Geometry: final body of the model. Coordinates: model frame, mm. Face numbers are marked on the shaded views. A direction names the side the tool comes from. Give positions to 0.01 mm unless a question says otherwise; leave off trailing zeros. Write each loop counter-clockwise with the first axis right and the second up, starting at its lowest first coordinate (ties: lowest second). Pieces come first, ordered by that corner, then holes. Notation, with made-up numbers: (2, 74) - (43, 74) arc R18 cw to (43, 98) - close; hole circle Ø8 at (46, 10.25). An arc over 180 degrees is marked (long way). Use CSV: the item, a comma, the result in double quotes. Start each with the question number.
(1) Section A-A on z = 1. Output: boundary loops of the cut face in (x, y), and give its area (3 significant figures).
(2) Reachability of the marked faces 5 and 6 from +Z, -Z, +X, -X, +Y, -Y: full face, straight path, thin tool, end or side. Return the list, or none.
(3) Section D-D on z = 6.25. Output: boundary loops of the cut face in (x, y), and give its area (3 significant figures).
(4) Draft query along Y for the marked faces 1, 2, 3 and 4. Return one class per face: released by +Y, released by -Y, zero draft, split by the parting line, or undercut.
(5) Line query: probe 1 along Y at (x, z) = (-20.5, 1.65); probe 2 along Y at (x, z) = (20.5, 7); probe 3 along Z at (x, y) = (16.5, 17.5). Output: solid intervals per line, ascending. Write a range as [from, to].
(6) Section C-C on y = 19.5. Output: boundary loops of the cut face in (x, z).
(7) First-contact query: pin 1 Ø4 at (x, y) = (-20.5, 19.5) entering from -Z; pin 2 Ø8.5 at (x, y) = (-20.5, 19.5) entering from +Z. Flat tips, straight axial feed; report the tip coordinate or a pass-through.
(8) Section B-B on x = 0. Output: boundary loops of the cut face in (y, z).
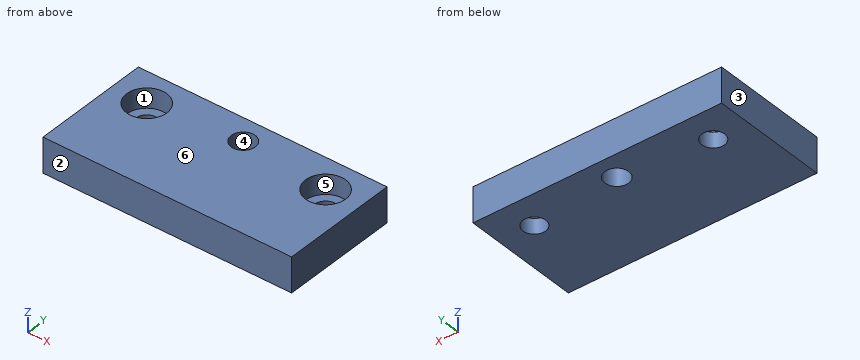
from build123d import *

# Parameters (mm, degrees)
F0_W     = 57
F0_H     = 27
F1_DEPTH = 8
F2_R     = 2.75
F2_R_2   = 2.6
F3_DEPTH = 9
F2_R_3   = 4.6
F4_DEPTH = 4.5


with BuildPart() as f1:
    # F0 (on Top) → F1 (new body)
    with BuildSketch(Plane.XY):
        with Locations((0, 13.5)):
            Rectangle(F0_W, F0_H)
    extrude(amount=F1_DEPTH)

    # F2 (on face) → F3 (cut)
    with BuildSketch(Plane.XY.offset(8)):
        with Locations((0, 21.5)):
            Circle(F2_R)
        with Locations((20.5, 19.5)):
            Circle(F2_R_2)
        with Locations((-20.5, 19.5)):
            Circle(F2_R_2)
    extrude(amount=-F3_DEPTH, mode=Mode.SUBTRACT)

    # F2 (on face) → F4 (cut)
    with BuildSketch(Plane.XY.offset(8)):
        with Locations((-20.5, 19.5)):
            Circle(F2_R_3)
        with Locations((-20.5, 19.5)):
            Circle(F2_R_2, mode=Mode.SUBTRACT)
        with Locations((20.5, 19.5)):
            Circle(F2_R_3)
        with Locations((20.5, 19.5)):
            Circle(F2_R_2, mode=Mode.SUBTRACT)
        with Locations((0, 21.5)):
            Circle(F2_R)
    extrude(amount=-F4_DEPTH, mode=Mode.SUBTRACT)


solid = f1.part
Check values:
1,outline,"(-28.5, 0) - (28.5, 0) - (28.5, 27) - (-28.5, 27) - close; hole circle Ø5.2 at (-20.5, 19.5); hole circle Ø5.5 at (0, 21.5); hole circle Ø5.2 at (20.5, 19.5)"
1,area,"1,470 mm²"
2,face 5,"+Z"
2,face 6,"+Z, +X, -X, +Y, -Y"
3,outline,"(-28.5, 0) - (28.5, 0) - (28.5, 27) - (-28.5, 27) - close; hole circle Ø9.2 at (-20.5, 19.5); hole circle Ø5.5 at (0, 21.5); hole circle Ø9.2 at (20.5, 19.5)"
3,area,"1,380 mm²"
4,face 1,"undercut"
4,face 2,"released by -Y"
4,face 3,"zero draft"
4,face 4,"undercut"
5,probe 1,"y = [0, 16.9], [22.1, 27]"
5,probe 2,"y = [0, 14.9], [24.1, 27]"
5,probe 3,"z = [0, 3.5]"
6,outline,"(-28.5, 0) - (-23.1, 0) - (-23.1, 3.5) - (-25.1, 3.5) - (-25.1, 8) - (-28.5, 8) - close; (-17.9, 0) - (-1.89, 0) - (-1.89, 8) - (-15.9, 8) - (-15.9, 3.5) - (-17.9, 3.5) - close; (1.89, 0) - (17.9, 0) - (17.9, 3.5) - (15.9, 3.5) - (15.9, 8) - (1.89, 8) - close; (23.1, 0) - (28.5, 0) - (28.5, 8) - (25.1, 8) - (25.1, 3.5) - (23.1, 3.5) - close"
7,pin 1,"passes through"
7,pin 2,"stops at z = 3.5"
8,outline,"(0, 0) - (18.75, 0) - (18.75, 8) - (0, 8) - close; (24.25, 0) - (27, 0) - (27, 8) - (24.25, 8) - close"
